```python
from build123d import *

# Parameters (mm, degrees)
SKETCH1_W           = 115
SKETCH1_H           = 73.849129594
SKETCH1_R           = 1.75
SKETCH1_W_2         = 16
SKETCH1_H_2         = 3.2
SKETCH1_W_3         = 3.2
SKETCH1_H_3         = 16
BOSS_EXTRUDE1_DEPTH = 3
FILLET1_R           = 5


with BuildPart() as part:
    # Sketch1 → Boss-Extrude1 (new body)
    with BuildSketch(Plane(origin=(0, 0, 0), x_dir=(1, 0, 0), z_dir=(0, 1, 0))):
        Rectangle(SKETCH1_W, SKETCH1_H)
        with Locations(Location((-42.5, 24.25, 0), (0, 0, 270))):
            Circle(SKETCH1_R, mode=Mode.SUBTRACT)
        with Locations(Location((42.5, 24.25, 0), (0, 0, 270))):
            Circle(SKETCH1_R, mode=Mode.SUBTRACT)
        with Locations(Location((-42.5, -24.25, 0), (0, 0, 270))):
            Circle(SKETCH1_R, mode=Mode.SUBTRACT)
        with Locations(Location((42.5, -24.25, 0), (0, 0, 270))):
            Circle(SKETCH1_R, mode=Mode.SUBTRACT)
        with Locations((-28, 31.6)):
            Rectangle(SKETCH1_W_2, SKETCH1_H_2, mode=Mode.SUBTRACT)
        with Locations((28, 31.6)):
            Rectangle(SKETCH1_W_2, SKETCH1_H_2, mode=Mode.SUBTRACT)
        with Locations((-50.1, 14)):
            Rectangle(SKETCH1_W_3, SKETCH1_H_3, mode=Mode.SUBTRACT)
        with Locations((-50.1, -14)):
            Rectangle(SKETCH1_W_3, SKETCH1_H_3, mode=Mode.SUBTRACT)
        with Locations((0, 31.6)):
            Rectangle(SKETCH1_W_2, SKETCH1_H_2, mode=Mode.SUBTRACT)
        with Locations((-28, -31.6)):
            Rectangle(SKETCH1_W_2, SKETCH1_H_2, mode=Mode.SUBTRACT)
        with Locations((28, -31.6)):
            Rectangle(SKETCH1_W_2, SKETCH1_H_2, mode=Mode.SUBTRACT)
        with Locations((0, -31.6)):
            Rectangle(SKETCH1_W_2, SKETCH1_H_2, mode=Mode.SUBTRACT)
        with Locations((50.1, -14)):
            Rectangle(SKETCH1_W_3, SKETCH1_H_3, mode=Mode.SUBTRACT)
        with Locations((50.1, 14)):
            Rectangle(SKETCH1_W_3, SKETCH1_H_3, mode=Mode.SUBTRACT)
    extrude(amount=BOSS_EXTRUDE1_DEPTH)

    # Fillet1
    fillet1_edges = [part.edges().sort_by_distance(p)[0] for p in [
        (57.5, 1.5, 36.924564797),
        (-57.5, 1.5, 36.924564797),
        (-57.5, 1.5, -36.924564797),
        (57.5, 1.5, -36.924564797),
    ]]
    fillet(fillet1_edges, radius=FILLET1_R)


solid = part.part
```
Source: CAD feature listing. Evaluate the final solid. Frame: model axes, mm. A direction names the side the tool comes from. Round coordinates to 2 decimals unless told otherwise and drop trailing zeros. Write each loop counter-clockwise with the first axis right and the second up, starting at its lowest first coordinate (ties: lowest second). Pieces come first, ordered by that corner, then holes. Notation, with made-up numbers: M 76.25,38 L 85.25,38 A27 ccw 85.25,76 Z; hole C 58,37.5 d2. An arc over 180 degrees is marked long. Answer as a JSON object with one key per item and string values. Group by question number.
(1) Section query C-C on y = 1. State how many separate pieces and enclosed holes the cut face has, then the cut area to 3 significant figures.
(2) Mould query, pull axis X, two halves, no side actions, for faces 3 (the flat face through (-1, 1, -36.925)), 4 (the flat face through (-50, 1, 6)), 5 (the flat face through (57.5, 1, 0)), 6 (the cylindrical face through (-56.074, 1.521, 35.421)). Classes: +X half, -X half, draft (parallel to the pull), parting line (faces both ways), or undercut.
(3) Ray query, line 1 (Z direction, x = 20.5, y = 1.8); line 2 (X direction, y = 1.3, z = -24.25); line 3 (X direction, y = 1.6, z = 6.5). Return the intervals inside material, ascending. Write a range as [from, to].
(4) Section query A-A on z = -24.25. Output: boundary loops of the cut face in (x, y).
(5) First-contact query: pin 1 (5.5 mm diameter, centred on x = -42.5, z = 24.25, fed in from +Y). Flat tip, straight axial feed; report the tip coordinate or a pass-through.
(6) Reachability of faces 1 (the flat face through (50, 1, -22)), 2 (the cylindrical face through (-56.074, 1.521, -35.421)) from +Z, -Z, +X, -X, +Y, -Y: full face, straight path, thin tool, end or side. Return the list, or none.
(7) Section query B-B on x = 42.5. Output: boundary loops of the cut face in (y, z).
Computed values:
{
 "1": {"separate pieces": "1", "enclosed holes": "14", "area": "7,920 mm^2"},
 "2": {"face 3": "draft", "face 4": "undercut", "face 5": "+X half", "face 6": "-X half"},
 "3": {"line 1": "[-36.92, -33.2], [-30, 30], [33.2, 36.92]", "line 2": "[-57.5, -44.25], [-40.75, 40.75], [44.25, 57.5]", "line 3": "[-57.5, -51.7], [-48.5, 48.5], [51.7, 57.5]"},
 "4": {"outline": "M -57.5,0 L -44.25,0 L -44.25,3 L -57.5,3 Z; M -40.75,0 L 40.75,0 L 40.75,3 L -40.75,3 Z; M 44.25,0 L 57.5,0 L 57.5,3 L 44.25,3 Z"},
 "5": {"pin 1": "y = 3"},
 "6": {"face 1": "+Y, -Y", "face 2": "-Z, -X, +Y, -Y"},
 "7": {"outline": "M 0,-36.92 L 3,-36.92 L 3,-26 L 0,-26 Z; M 0,-22.5 L 3,-22.5 L 3,22.5 L 0,22.5 Z; M 0,26 L 3,26 L 3,36.92 L 0,36.92 Z"}
}
